Autodesk Inventor part; units mm, degrees
ref_plane "YZ Plane" through (0, 0, 0) normal (1, 0, 0) x (0, 1, 0)
ref_plane "XZ Plane" through (0, 0, 0) normal (0, 1, 0) x (-1, 0, 0)
ref_plane "XY Plane" through (0, 0, 0) normal (0, 0, 1) x (1, 0, 0)
sketch "Sketch1" plane through (0, 0, 0) normal (0, 0, 1) x (1, 0, 0)
  arc A0 (-39.1074, 3.3431) -> (-3.3431, 39.1074) centre (0, 0) ccw
  line L0 (0, 0) -> (30.017, 0) construction
  line L1 (-39.1074, 3.3431) -> (-3.3431, 39.1074)
  line L2 (0, 0) -> (39.25, 0) construction
  circle A1 centre (22.8042, -22.8042) radius 3
  circle A2 centre (-26.9378, -17.7318) radius 3
  circle A3 centre (17.7318, 26.9378) radius 3
  dimension "d0" = 78.5
  dimension "d6" = 6
  dimension "d9" = 6
  dimension "d10" = 6
extrude "Extrusion1" add sketch "Sketch1" along normal blind 10
sketch "Sketch2" plane through (0, 0, 10) normal (0, 0, 1) x (1, 0, 0)
  circle A0 centre (17.7318, 26.9378) radius 3
  circle A1 centre (17.7318, 26.9378) radius 5
  circle A2 centre (22.8042, -22.8042) radius 3
  circle A3 centre (22.8042, -22.8042) radius 5
  circle A4 centre (-26.9378, -17.7318) radius 3
  circle A5 centre (-26.9378, -17.7318) radius 5
  point P0 (0, 0)
  dimension "d13" = 10
  dimension "d14" = 10
  dimension "d15" = 10
extrude "Extrusion2" cut sketch "Sketch2" against normal blind 5 contours A1
extrude "Extrusion3" cut sketch "Sketch2" against normal blind 5 contours A5
extrude "Extrusion4" cut sketch "Sketch2" against normal blind 5 contours A3
sketch "Sketch3" plane through (0, 0, 10) normal (0, 0, 1) x (1, 0, 0)
  line L0 (0, 0) -> (25, 0) construction
  circle A0 centre (-12.5, -21.6506) radius 2
  arc A1 (-39.1074, 3.3431) -> (-3.3431, 39.1074) centre (0, 0) ccw
  circle A2 centre (25, 0) radius 2
  circle A3 centre (-12.5, 21.6506) radius 2
  dimension "d24" = 4
  dimension "d27" = 360
extrude "Extrusion5" cut sketch "Sketch3" against normal through all contours A0
extrude "Extrusion6" cut sketch "Sketch3" against normal through all contours A2
extrude "Extrusion7" cut sketch "Sketch3" against normal through all contours A3
sketch "Sketch5" plane through (0, 0, 10) normal (0, 0, 1) x (1, 0, 0)
  circle A0 centre (17.7318, 26.9378) radius 3
  circle A1 centre (22.8042, -22.8042) radius 3
  circle A2 centre (-26.9378, -17.7318) radius 5
  arc A3 (-39.1074, 3.3431) -> (-3.3431, 39.1074) centre (0, 0) ccw
  arc A4 (-30.0025, -6.3107) -> (-23.4023, -14.1962) centre (17.7318, 26.9378) ccw
  line L0 (-38.9658, -4.7151) -> (-34.7002, -4.204)
  line L1 (-24.2556, -21.9514) -> (-29.8381, -25.5)
  circle A5 centre (-26.9378, -17.7318) radius 5
  arc A6 (-30.0025, -6.3107) -> (-34.7002, -4.204) centre (-34.1053, -9.1685) ccw
  arc A7 (12.2473, -17.7267) -> (22.2969, -17.83) centre (17.7318, 26.9378) ccw
  arc A8 (11.0285, -27.6521) -> (23.3114, -27.7784) centre (17.7318, 26.9378) ccw
  circle A9 centre (22.8042, -22.8042) radius 5
extrude "Extrusion11" cut sketch "Sketch5" against normal blind 5 contours A2 L1 A3 L0 A6 A4
sketch "Sketch6" plane through (0, 0, 5) normal (0, 0, 1) x (1, 0, 0)
  circle A0 centre (17.7318, 26.9378) radius 3
  circle A1 centre (22.8042, -22.8042) radius 3
  circle A2 centre (-26.9378, -17.7318) radius 3
  arc A3 (12.0035, -19.7118) -> (22.4998, -19.8197) centre (17.7318, 26.9378) ccw
  arc A4 (11.2723, -25.6671) -> (23.1085, -25.7887) centre (17.7318, 26.9378) ccw
  arc A5 (12.2473, -17.7267) -> (11.0285, -27.6521) centre (11.6379, -22.6894) ccw
  arc A6 (12.0035, -19.7118) -> (11.2723, -25.6671) centre (11.6379, -22.6894) ccw
  arc A7 (-31.6436, -7.4538) -> (-24.8165, -15.6104) centre (17.7318, 26.9378) ccw
  arc A8 (-36.567, -10.8831) -> (-29.0592, -19.8531) centre (17.7318, 26.9378) ccw
  arc A9 (-30.0025, -6.3107) -> (-34.7002, -4.204) centre (-34.1053, -9.1685) ccw
  arc A10 (-31.6436, -7.4538) -> (-36.567, -10.8831) centre (-34.1053, -9.1685) ccw
  point P0 (0, 0)
  dimension "d69" = 106
  dimension "d70" = 6
  dimension "d71" = 6
extrude "Extrusion14" cut sketch "Sketch6" against normal blind 5 contours A2 | A2 A8 A10 A7
sketch "Sketch7" plane through (0, 0, 10) normal (0, 0, 1) x (1, 0, 0)
  line L0 (-3.3431, 39.1074) -> (-39.1074, 3.3431)
  arc A0 (-29.8381, -25.5) -> (-3.3431, 39.1074) centre (0, 0) ccw
  line L1 (-2.5781, 39.1652) -> (-39.1652, 2.5781)
  line L2 (-2.5781, 39.1652) -> (49.1639, 39.1652) construction
  arc A1 (-39.1074, 3.3431) -> (-38.9658, -4.7151) centre (0, 0) ccw
  dimension "d77" = 135
extrude "Extrusion15" cut sketch "Sketch7" against normal blind 10
sketch "Sketch8" plane through (0, 0, 10) normal (0, 0, 1) x (1, 0, 0)
  circle A0 centre (17.7318, 26.9378) radius 3
  line L0 (17.7318, 26.9378) -> (67.7318, 26.9378) construction
  circle A1 centre (22.8042, -22.8042) radius 3
  arc A2 (14.342, -17.9343) -> (13.5888, -27.9059) centre (13.9654, -22.9201) ccw
  arc A3 (14.342, -17.9343) -> (22.2969, -17.83) centre (17.7318, 26.9378) ccw
  arc A4 (13.5888, -27.9059) -> (23.3114, -27.7784) centre (17.7318, 26.9378) ccw
  circle A5 centre (22.8042, -22.8042) radius 5
  point P0 (0, 0)
  dimension "d84" = 10
  dimension "d87" = 10
extrude "Extrusion16" cut sketch "Sketch8" against normal blind 5 contours A3 A5 A4 A2 | A5
sketch "Sketch9" plane through (0, 0, 5) normal (0, 0, 1) x (1, 0, 0)
  arc A0 (14.342, -17.9343) -> (13.5888, -27.9059) centre (13.9654, -22.9201) ccw
  arc A1 (14.1914, -19.9286) -> (13.7394, -25.9116) centre (13.9654, -22.9201) ccw
  circle A2 centre (17.7318, 26.9378) radius 3
  circle A3 centre (22.8042, -22.8042) radius 3
  arc A4 (14.1914, -19.9286) -> (22.4998, -19.8197) centre (17.7318, 26.9378) ccw
  arc A5 (13.7394, -25.9116) -> (23.1085, -25.7887) centre (17.7318, 26.9378) ccw
  point P0 (0, 0)
  dimension "d90" = 6
  dimension "d92" = 6
extrude "Extrusion17" cut sketch "Sketch9" against normal blind 5 contours A4 A3 A5 A1
thread "Thread1"
thread "Thread2"
thread "Thread3"
properties part number "Encoder Mount Base" material "ABS Plastic"
Geometry check sheet. Reference: the model listing, model coordinates, mm. A direction names the side the tool comes from. Give positions to 0.01 mm unless a question says otherwise; leave off trailing zeros. Loops run counter-clockwise (first coordinate to the right, second up) from the corner with the lowest first, then second, coordinate; pieces in that order, holes last. Notation, with made-up numbers: (-26.5, -13.75) -> (16.5, -13.75) arc R7 ccw to (16.5, -9.75) -> close; hole circle Ø7 at (-12, 77.5). An arc over 180 degrees is marked (long way). Answer in a Markdown table with one row per item. Add a question column.
1) Gauge pin test, flat ends, axial feed: P1, Ø3, axis at x = 18.5, y = 25.5, coming from the +Z side; P2, Ø2, axis at y = 13, z = 2.5, coming from the +X side; P3, Ø4, axis at x = 2.5, z = 5, coming from the +Y side. Record the tip position at first contact, or that the pin passes through.
2) Cross-section at D-D on x = 19. Record the boundary of the cut face in (y, z).
3) Set-up check for faces 1 (the face through (18.3, -26.3, 5)), 2 (the face through (18.36, -26.06, 2.54)), 3 (the face through (-32.025, -4.622, 7.535)): record each of +Z, -Z, +X, -X, +Y, -Y from which the full face is reachable in a straight line by a thin tool's end or side.
4) Cross-section at B-B on y = 0. Record the boundary of the cut face in (x, z).
5) Cross-section at C-C on z = 7. Record the boundary of the cut face in (x, y).
6) Cross-section at A-A on x = -12.5. Record the boundary of the cut face in (y, z), and give its area (3 significant figures).
7) Material ranges on probe 1 along X at (y, z) = (-20, 6.75); probe 2 along Y at (x, z) = (25.5, 4.25); probe 3 along Y at (x, z) = (-12, 3), recorded low to high. Write a range as from..to.
8) Draft check along X on faces 4 (the face through (-21.975, -18.341, 7.535)), 5 (the face through (-36.863, -4.463, 7.535)), 6 (the face through (28.679, -26.797, 4.93)). Enter one of: pulls with the +X half, pulls with the -X half, needs draft (parallel to the pull), parting line crosses it, or undercut.
Outcome:
| question | item | result |
|---|---|---|
| 1 | P1 | stops at z = 5 |
| 1 | P2 | stops at x = 37.37 |
| 1 | P3 | stops at y = 39.25 |
| 2 | outline | (-34.34, 0) -> (-26.05, 0) -> (-26.05, 5) -> (-28.05, 5) -> (-28.05, 10) -> (-34.34, 10) -> close; (-20.05, 0) -> (24.22, 0) -> (24.22, 5) -> (22.1, 5) -> (22.1, 10) -> (-18.04, 10) -> (-18.04, 5) -> (-20.05, 5) -> close; (29.66, 0) -> (34.34, 0) -> (34.34, 10) -> (31.77, 10) -> (31.77, 5) -> (29.66, 5) -> close |
| 3 | face 1 | +Z |
| 3 | face 2 | +Z, -Z |
| 3 | face 3 | +Z, -Y |
| 4 | outline | (-39.25, 0) -> (23, 0) -> (23, 10) -> (-39.25, 10) -> close; (27, 0) -> (39.25, 0) -> (39.25, 10) -> (27, 10) -> close |
| 5 | outline | (-39.17, 2.58) arc R39.25 ccw to (-38.97, -4.72) -> (-34.7, -4.2) arc R5 cw to (-30, -6.31) arc R58.17 ccw to (-23.4, -14.2) arc R5 cw to (-24.26, -21.95) -> (-29.84, -25.5) arc R39.25 ccw (long way) to (-2.58, 39.17) -> close; hole circle Ø4 at (-12.5, -21.65); hole circle Ø4 at (-12.5, 21.65); hole circle Ø10 at (17.73, 26.94); hole (13.59, -27.91) arc R55 ccw to (23.31, -27.78) arc R5 ccw to (22.3, -17.83) arc R45 cw to (14.34, -17.93) arc R5 ccw to start; hole circle Ø4 at (25, 0) |
| 6 | outline | (-37.21, 0) -> (-23.65, 0) -> (-23.65, 10) -> (-37.21, 10) -> close; (-19.65, 0) -> (19.65, 0) -> (19.65, 10) -> (-19.65, 10) -> close; (23.65, 0) -> (29.24, 0) -> (29.24, 10) -> (23.65, 10) -> close |
| 6 | area | 584 mm^2 |
| 7 | probe 1 | x = -22.48..-13.63, -11.37..9.91, 26.94..33.77 |
| 7 | probe 2 | y = -29.84..-24.12, -21.49..-1.94, 1.94..29.84 |
| 7 | probe 3 | y = -37.37..-23.59, -19.71..19.71, 23.59..29.74 |
| 8 | face 4 | pulls with the -X half |
| 8 | face 5 | undercut |
| 8 | face 6 | parting line crosses it |
